CAD build for the part. Positions are in the model's coordinates, mm. A direction names the side the tool comes from. Give positions to 0.01 mm unless a question says otherwise; leave off trailing zeros. Loops run counter-clockwise (first coordinate to the right, second up) from the corner with the lowest first, then second, coordinate; pieces in that order, holes last. Notation, with made-up numbers: M 28.25,-25 L 64.25,-25 A19 cw 64.25,-14 Z; hole C 80.5,-11.75 d1. An arc over 180 degrees is marked long. Answer as CSV lines item,"result".
Autodesk Inventor part; units mm, degrees
ref_plane "YZ Plane" through (0, 0, 0) normal (1, 0, 0) x (0, 1, 0)
ref_plane "XZ Plane" through (0, 0, 0) normal (0, 1, 0) x (-1, 0, 0)
ref_plane "XY Plane" through (0, 0, 0) normal (0, 0, 1) x (1, 0, 0)
sketch "Sketch1" plane through (0, 0, 0) normal (0, 0, 1) x (1, 0, 0)
  line L0 (-127.5242, -32.3587) -> (-188.9758, -32.3587)
  line L1 (-128.9881, -97.1287) -> (-187.5119, -97.1287)
  line L2 (-113.8, -97.1287) -> (-113.8, -85.5717)
  circle A0 centre (-120.15, -39.9787) radius 2.3114
  circle A1 centre (-120.15, -90.7787) radius 2.3114
  circle A2 centre (-170.95, -90.7787) radius 2.3114
  circle A3 centre (-170.95, -39.9787) radius 2.3114
  circle A4 centre (-158.25, -39.9787) radius 2.3114
  circle A5 centre (-158.25, -90.7787) radius 2.3114
  circle A6 centre (-120.15, -39.9787) radius 6.35
  circle A7 centre (-170.95, -39.9787) radius 6.35
  circle A8 centre (-170.95, -90.7787) radius 6.35
  circle A9 centre (-120.15, -90.7787) radius 6.35
  line L3 (-170.95, -33.6287) -> (-120.15, -33.6287)
  line L4 (-113.8, -39.9787) -> (-113.8, -90.7787)
  line L5 (-120.15, -97.1287) -> (-170.95, -97.1287)
  line L6 (-170.95, -46.3287) -> (-129.675, -46.3287)
  line L7 (-126.5, -49.5037) -> (-126.5, -81.2537)
  line L8 (-129.675, -84.4287) -> (-170.95, -84.4287)
  arc A10 (-126.5, -49.5037) -> (-129.675, -46.3287) centre (-129.675, -49.5037) ccw
  arc A11 (-129.675, -84.4287) -> (-126.5, -81.2537) centre (-129.675, -81.2537) ccw
  circle A12 centre (-170.95, -39.9787) radius 2.3114
  circle A13 centre (-120.15, -39.9787) radius 2.3114
  circle A14 centre (-120.15, -90.7787) radius 2.3114
  circle A15 centre (-170.95, -90.7787) radius 2.3114
  circle A16 centre (-158.25, -90.7787) radius 2.3114
  circle A17 centre (-158.25, -39.9787) radius 2.3114
  point P0 (0, 0)
  dimension "d6" = 12.7
  dimension "d7" = 12.7
  dimension "d8" = 12.7
  dimension "d9" = 12.7
  dimension "d10" = 3.175
extrude "Extrusion1" add sketch "Sketch1" along normal blind 1.5875
sketch "Sketch2" plane through (0, 0, 1.5875) normal (0, 0, 1) x (1, 0, 0)
  circle A0 centre (-158.25, -39.9787) radius 2.3114
  circle A1 centre (-158.25, -39.9787) radius 2.3114
  circle A2 centre (-158.25, -90.7787) radius 2.3114
  circle A3 centre (-158.25, -90.7787) radius 2.3114
  circle A4 centre (-145.55, -90.7787) radius 2.3368
  circle A5 centre (-170.95, -90.7787) radius 2.3114
  circle A6 centre (-145.55, -39.9787) radius 2.3368
  circle A7 centre (-120.15, -65.3787) radius 2.3368
  circle A8 centre (-120.15, -39.9787) radius 2.3114
  line L0 (-113.8, -90.7787) -> (-113.8, -39.9787)
  circle A9 centre (-170.95, -39.9787) radius 2.3114
  circle A10 centre (-120.15, -90.7787) radius 2.3114
  point P0 (0, 0)
  dimension "d13" = 4.6736
  dimension "d14" = 25.4
  dimension "d15" = 4.6736
  dimension "d16" = 4.6736
  dimension "d17" = 25.4
  dimension "d18" = 6.35
  dimension "d23" = 25.4
  dimension "d24" = 25.4
  dimension "d25" = 25.4
extrude "Extrusion2" cut sketch "Sketch2" against normal blind 25.4 contours A4 | A6 | A7
extrude "Extrusion3" add sketch "Sketch2" against normal up to surface (1.5875 mm away) contours A0 | A2
equation "\"BendRadius\" = Thickness"
equation "\"BendReliefWidth\" = Thickness"
equation "\"BendReliefDepth\" = 0.5 * Thickness"
equation "\"CornerReliefSize\" = 4 * Thickness"
equation "\"MinimumRemnant\" = 2 * Thickness"
equation "\"TransitionRadius\" = BendRadius"
equation "\"JacobiRadiusSize\" = BendRadius"
equation "\"GapSize\" = Thickness"
properties part number "frontgusset" material "Polycarbonate, Clear"
1) Band-saw the part on C-C on z = 0.45. Give the cut face in (x, y) (3 decimals), and give its area (3 significant figures).
Answer below:
outline,"M -170.95,-97.129 L -120.15,-97.129 A6.35 ccw -113.8,-90.779 L -113.8,-39.979 A6.35 ccw -120.15,-33.629 L -170.95,-33.629 A6.35 ccw -170.95,-46.329 L -129.675,-46.329 A3.175 cw -126.5,-49.504 L -126.5,-81.254 A3.175 cw -129.675,-84.429 L -170.95,-84.429 A6.35 ccw Z; hole C -170.95,-90.779 d4.623; hole C -170.95,-39.979 d4.623; hole C -145.55,-90.779 d4.674; hole C -145.55,-39.979 d4.674; hole C -120.15,-65.379 d4.674; hole C -120.15,-90.779 d4.623; hole C -120.15,-39.979 d4.623"
area,"1,930 mm^2"
2) Band-saw the part on D-D on y = -53.5. Give the cut face in (x, z).
Answer below:
outline,"M -126.5,0 L -113.8,0 L -113.8,1.59 L -126.5,1.59 Z"
3) Which spindle directions (+Z, -Z, +X, -X, +Y, -Y) get a long thin tool onto all of the face, cutting with end or side? Do faces 4 (the face through (-151, -46.329, 1)), 5 (the face through (-147.404, -41.401, 0.805)). Say none if no direction does.
Answer below:
face 4,"+Z, -Z, -X"
face 5,"+Z, -Z"
4) Mould opens along Y. For faces 1 (the face through (-172.654, -92.341, 0.783)), 2 (the face through (-115.71, -35.44, 0.78)), 3 (the face through (-113.8, -65, 1)) say: +Y half, -Y half, draft (parallel to the pull), parting line (faces both ways), or undercut.
Answer below:
face 1,"undercut"
face 2,"+Y half"
face 3,"draft"
5) Band-saw the part on B-B on x = -155.5. Give the cut face in (y, z).
Answer below:
outline,"M -97.13,0 L -84.43,0 L -84.43,1.59 L -97.13,1.59 Z; M -46.33,0 L -33.63,0 L -33.63,1.59 L -46.33,1.59 Z"
6) Band-saw the part on A-A on x = -145.55. Give the cut face in (y, z).
Answer below:
outline,"M -97.13,0 L -93.12,0 L -93.12,1.59 L -97.13,1.59 Z; M -88.44,0 L -84.43,0 L -84.43,1.59 L -88.44,1.59 Z; M -46.33,0 L -42.32,0 L -42.32,1.59 L -46.33,1.59 Z; M -37.64,0 L -33.63,0 L -33.63,1.59 L -37.64,1.59 Z"
7) Drill centre lines: line 1 (Y direction, x = -120.15, z = 1.15); line 2 (Y direction, x = -165.5, z = 0.75); line 3 (X direction, y = -90, z = 1.35). Where is each one in solid material? Low to high. Write a range as from..to.
Answer below:
line 1,"y = -97.13..-93.09, -88.47..-67.72, -63.04..-42.29, -37.67..-33.63"
line 2,"y = -97.13..-84.43, -46.33..-33.63"
line 3,"x = -177.25..-173.13, -168.77..-147.75, -143.35..-122.33, -117.97..-113.8"
8) Flat gauge pins, fed straight in: pin 1 (3 mm diameter, centred on x = -120.15, y = -65.38, fed in from +Z); pin 2 (7.5 mm diameter, centred on x = -145.55, y = -39.98, fed in from +Z). Where does each tip first touch, or does it go through?
Answer below:
pin 1,"passes through"
pin 2,"stops at z = 1.59"
